from build123d import *

# Parameters (mm, degrees)
SKETCH_R        = 28.75
PAD_DEPTH       = 50
SKETCH001_R     = 24
POCKET_DEPTH    = 50
CHAMFER_SIZE    = 4
CHAMFER001_SIZE = 1


with BuildPart() as part:
    # Sketch → Pad (new body)
    with BuildSketch(Plane.XY):
        Circle(SKETCH_R)
    extrude(amount=PAD_DEPTH)

    # Sketch001 (on Face3 of Pad) → Pocket (cut)
    with BuildSketch(Plane.XY.offset(50)):
        Circle(SKETCH001_R)
    extrude(amount=-POCKET_DEPTH, mode=Mode.SUBTRACT)

    # Chamfer
    chamfer_edges = [part.edges().sort_by_distance(p)[0] for p in [
        (-28.75, 0, 50),
    ]]
    chamfer(chamfer_edges, length=CHAMFER_SIZE)

    # Chamfer001
    chamfer001_edges = [part.edges().sort_by_distance(p)[0] for p in [
        (-28.75, 0, 0),
    ]]
    chamfer(chamfer001_edges, length=CHAMFER001_SIZE)


solid = part.part
Model file for the job. Use its own axes, mm. Give positions to 0.01 mm unless a question says otherwise; leave off trailing zeros. Write each loop counter-clockwise with the first axis right and the second up, starting at its lowest first coordinate (ties: lowest second). Pieces come first, ordered by that corner, then holes. Notation, with made-up numbers: M -22.75,44.25 L -6.75,44.25 A32 cw -6.75,79.25 Z; hole C 30.5,1.25 d4. An arc over 180 degrees is marked long. One line per item, written item: value. Start each with the question number.
Q1. Two-plate mould, pull along Y, no slides. Class faces 1 (the cylindrical face through (-23.977, 1.055, 25.35)), 2 (the flat face through (-4, 24, 50)), 3 (the conical face through (-5.407, -24.351, 49.806)): +Y half, -Y half, draft (parallel to the pull), parting line (faces both ways), or undercut.
Q2. Saw through at A-A, the plane y = 0. Write the cut outline in (x, z).
Q3. Probe probe 1 along Y at (x, z) = (0, 24); probe 2 along Y at (x, z) = (15.5, 46.5); probe 3 along X at (y, z) = (-9, 45) (3 decimals). List the from-to ranges inside material, lowest first. Write a range as [from, to].
Q4. Saw through at C-C, the plane z = 19.5. Write the cut outline in (x, y).
Q5. Drop flat-ended pins along their axis: pin 1 Ø8 at (x, z) = (14, 31.5) entering from +Y; pin 2 Ø12 at (y, z) = (1, 36) entering from +X; pin 3 Ø10 at (y, z) = (-17.5, 18.5) entering from +X; pin 4 Ø6 at (x, z) = (9, 36) entering from +Y. Give the stop position or say it passes through.
Output values:
1. face 1: undercut
1. face 2: draft
1. face 3: parting line
2. outline: M -28.75,1 L -27.75,0 L -24,0 L -24,50 L -24.75,50 L -28.75,46 Z; M 24,0 L 27.75,0 L 28.75,1 L 28.75,46 L 24.75,50 L 24,50 Z
3. probe 1: y = [-28.75, -24], [24, 28.75]
3. probe 2: y = [-23.62, -18.32], [18.32, 23.62]
3. probe 3: x = [-27.305, -22.249], [22.249, 27.305]
4. outline: C 0,0 d57.5; hole C 0,0 d48
5. pin 1: stops at y = 26.95
5. pin 2: stops at x = 28.75
5. pin 3: stops at x = 25.89
5. pin 4: stops at y = 28.12
